The listing builds one solid part. Answer for the finished solid, in the listing's coordinates (mm). Face numbers are marked on the shaded views. A direction names the side the tool comes from. Give positions to 0.01 mm unless a question says otherwise; leave off trailing zeros. Order: outer loops, then holes, each group sorted by start corner. A loop starts at its lowest first (then second) coordinate and runs counter-clockwise, first axis right, second up. Notation, with made-up numbers: (-4.75, 66.5) - (15.25, 66.5) arc R14 cw to (15.25, 79.5) - close; hole circle Ø10 at (-35, 59). An arc over 180 degrees is marked (long way). Write each question's results on one line, items separated by ' | '. Start each with the question number.
1. Section D-D (y = 0) is taken. State how many separate pieces and enclosed holes the cut face has, and give its area (3 significant figures).
2. Which of the six approach directions +Z, -Z, +X, -X, +Y, -Y give full straight-line access (tool end or side, diameter ignored) to the marked faces 4, 5 and 6?
3. Section A-A (z = 88.5) is taken. Give the vertices of the cut face in (x, y).
4. Determine the mould class of the marked faces 1, 2 and 3 for opening direction X: released by +X, released by -X, zero draft, split by the parting line, or undercut.
5. Flat-ended cylindrical pins translate along their axes: pin 1 (2 mm diameter, centred on x = -16, z = 72.5, fed in from +Y); pin 2 (4.5 mm diameter, centred on x = -15.71, z = 73.6, fed in from -Y); pin 3 (5 mm diameter, centred on x = -0.5, z = 72.5, fed in from -Y); pin 4 (1 mm diameter, centred on x = 3, y = 0.5, fed in from -Z). Find the tip coordinate at first contact, or state that the pin passes through.
6. Find the intervals of material crossed by L1, parallel to X at y = -5.5, z = 75 (3 decimals); L2, parallel to Y at x = 2.5, z = 74.5; L3, parallel to Z at x = -2.5, y = -33, in increasing order.
7. Section C-C (y = -14.5) is taken. Give the vertices of the cut face in (x, z), and give its area (3 significant figures).
8. Section B-B (x = 16) is taken. Give the vertices of the cut face in (y, z), and give its area (3 significant figures).
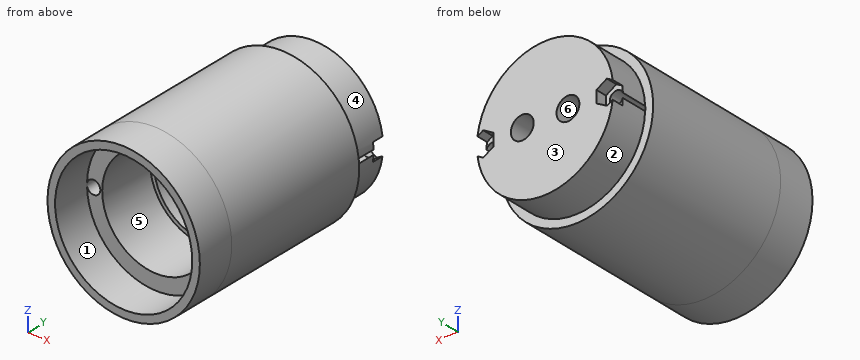
from build123d import *

# Parameters (mm, degrees)
SKETCH1_R               = 17.9
BOSS_EXTRUDE1_DEPTH     = 10
SKETCH2_R               = 20
BOSS_EXTRUDE2_DEPTH     = 40
SKETCH3_R               = 1.75
CUT_EXTRUDE1_DEPTH      = 1
CUT_EXTRUDE1_DEPTH_BACK = 119
CUT_EXTRUDE2_DEPTH      = 3
CUT_EXTRUDE4_START      = -10
SKETCH5_R               = 12
CUT_EXTRUDE4_DEPTH      = 43
FILLET1_R               = 10
SKETCH6_R               = 20
SKETCH6_R_2             = 18
BOSS_EXTRUDE3_DEPTH     = 10
SKETCH7_R               = 13
CUT_EXTRUDE5_DEPTH      = 40
FILLET2_R               = 10
SKETCH8_R               = 3
CUT_EXTRUDE6_DEPTH      = 11
CUT_EXTRUDE6_DEPTH_BACK = 51
SKETCH10_R              = 14
CUT_EXTRUDE7_DEPTH      = 15


with BuildPart() as part:
    # Sketch1 → Boss-Extrude1 (new body)
    with BuildSketch(Plane(origin=(0, 13.694359, 0), x_dir=(-1, 0, 0), z_dir=(0, -1, 0))):
        with Locations((-0.536003, -73.600817)):
            Circle(SKETCH1_R)
    extrude(amount=BOSS_EXTRUDE1_DEPTH)

    # Sketch2 → Boss-Extrude2 (add)
    with BuildSketch(Plane(origin=(0, 3.694359, 0), x_dir=(-1, 0, 0), z_dir=(0, -1, 0))):
        with Locations((-0.536003, -73.600817)):
            Circle(SKETCH2_R)
    extrude(amount=BOSS_EXTRUDE2_DEPTH)

    # Sketch3 → Cut-Extrude1 (cut, two sides)
    with BuildSketch(Plane(origin=(0, 81.694359, 0), x_dir=(1, 0, 0), z_dir=(0, 1, 0))) as cut_extrude1_sk:
        with Locations((-15.713997, -73.600817)):
            Circle(SKETCH3_R)
        with Locations((16.786003, -73.600817)):
            Circle(SKETCH3_R)
    extrude(amount=CUT_EXTRUDE1_DEPTH, mode=Mode.SUBTRACT)
    extrude(cut_extrude1_sk.sketch, amount=-CUT_EXTRUDE1_DEPTH_BACK, mode=Mode.SUBTRACT)

    # Sketch4 → Cut-Extrude2 (cut)
    with BuildSketch(Plane(origin=(0, 13.694359, 0), x_dir=(1, 0, 0), z_dir=(0, 1, 0))):
        Polygon((-15.759938, -70.425723), (-18.48668, -72.053056), (-18.440739, -75.22815), (-15.668056, -76.775911), (-12.941314, -75.148578), (-12.987255, -71.973484), align=None)
        Polygon((16.786003, -70.42539), (14.036003, -72.013104), (14.036003, -75.18853), (16.786003, -76.776243), (19.536003, -75.18853), (19.536003, -72.013104), align=None)
    extrude(amount=-CUT_EXTRUDE2_DEPTH, mode=Mode.SUBTRACT)

    # Sketch5 → Cut-Extrude4 (cut)
    with BuildSketch(Plane(origin=(0, 13.694359, 0), x_dir=(1, 0, 0), z_dir=(0, 1, 0)).offset(CUT_EXTRUDE4_START)):
        with Locations((0.536003, -73.600817)):
            Circle(SKETCH5_R)
    extrude(amount=-CUT_EXTRUDE4_DEPTH, mode=Mode.SUBTRACT)

    # Fillet1
    fillet1_edges = [part.edges().sort_by_distance(p)[0] for p in [
        (-11.463997, 3.694359, 73.600817),
    ]]
    fillet(fillet1_edges, radius=FILLET1_R)

    # Sketch6 → Boss-Extrude3 (add)
    with BuildSketch(Plane.XZ.offset(36.305641)):
        with Locations((0.536003, 73.600817)):
            Circle(SKETCH6_R)
        with Locations((0.536003, 73.600817)):
            Circle(SKETCH6_R_2, mode=Mode.SUBTRACT)
    extrude(amount=BOSS_EXTRUDE3_DEPTH)

    # Sketch7 → Cut-Extrude5 (cut)
    with BuildSketch(Plane(origin=(0, -36.305641, 0), x_dir=(-1, 0, 0), z_dir=(0, -1, 0))):
        with Locations((-0.536003, -73.600817)):
            Circle(SKETCH7_R)
    extrude(amount=-CUT_EXTRUDE5_DEPTH, mode=Mode.SUBTRACT)

    # Fillet2
    fillet2_edges = [part.edges().sort_by_distance(p)[0] for p in [
        (13.536003, 3.694359, 73.600817),
    ]]
    fillet(fillet2_edges, radius=FILLET2_R)

    # Sketch8 → Cut-Extrude6 (cut, two sides)
    with BuildSketch(Plane(origin=(0, -36.305641, 0), x_dir=(-1, 0, 0), z_dir=(0, -1, 0))) as cut_extrude6_sk:
        with Locations((5.463997, -73.600817)):
            Circle(SKETCH8_R)
        with Locations((-6.536003, -73.600817)):
            Circle(SKETCH8_R)
    extrude(amount=CUT_EXTRUDE6_DEPTH, mode=Mode.SUBTRACT)
    extrude(cut_extrude6_sk.sketch, amount=-CUT_EXTRUDE6_DEPTH_BACK, mode=Mode.SUBTRACT)

    # Sketch10 → Cut-Extrude7 (cut)
    with BuildSketch(Plane(origin=(0, -36.305641, 0), x_dir=(-1, 0, 0), z_dir=(0, -1, 0))):
        with Locations((-0.536003, -73.600817)):
            Circle(SKETCH10_R)
    extrude(amount=-CUT_EXTRUDE7_DEPTH, mode=Mode.SUBTRACT)


solid = part.part
Reported:
1) separate pieces: 1 | enclosed holes: 3 | area: 874 mm²
2) face 4: +Z, +Y | face 5: -Y | face 6: +Y, -Y
3) outline: (-12.81, -46.31) - (-9.56, -46.31) - (-9.56, -36.31) - (10.64, -36.31) - (10.64, -46.31) - (13.88, -46.31) - (13.88, 3.69) - (10.46, 3.69) - (10.46, 13.69) - (-9.38, 13.69) - (-9.38, 3.69) - (-12.81, 3.69) - close
4) face 1: undercut | face 2: split by the parting line | face 3: zero draft
5) pin 1: y = 10.69 | pin 2: y = -46.31 | pin 3: y = 3.64 | pin 4: z = 53.7
6) L1: -19.415 to -16.765, -14.663 to -12.356, 13.428 to 15.735, 17.837 to 20.487 | L2: 3.69 to 13.69 | L3: 53.83 to 59.93, 87.27 to 93.37
7) outline: circle Ø40 at (0.54, 73.6); hole circle Ø3.5 at (-15.71, 73.6); hole circle Ø26 at (0.54, 73.6); hole circle Ø3.5 at (16.79, 73.6) | area: 706 mm²
8) outline: (-46.31, 60.92) - (3.69, 60.92) - (3.69, 64.59) - (13.69, 64.59) - (13.69, 70.88) - (10.69, 70.88) - (10.69, 72.04) - (-36.31, 72.04) - (-36.31, 64.39) - (-46.31, 64.39) - close; (-46.31, 82.81) - (-36.31, 82.81) - (-36.31, 75.16) - (10.69, 75.16) - (10.69, 76.32) - (13.69, 76.32) - (13.69, 82.62) - (3.69, 82.62) - (3.69, 86.28) - (-46.31, 86.28) - close | area: 1,100 mm²
